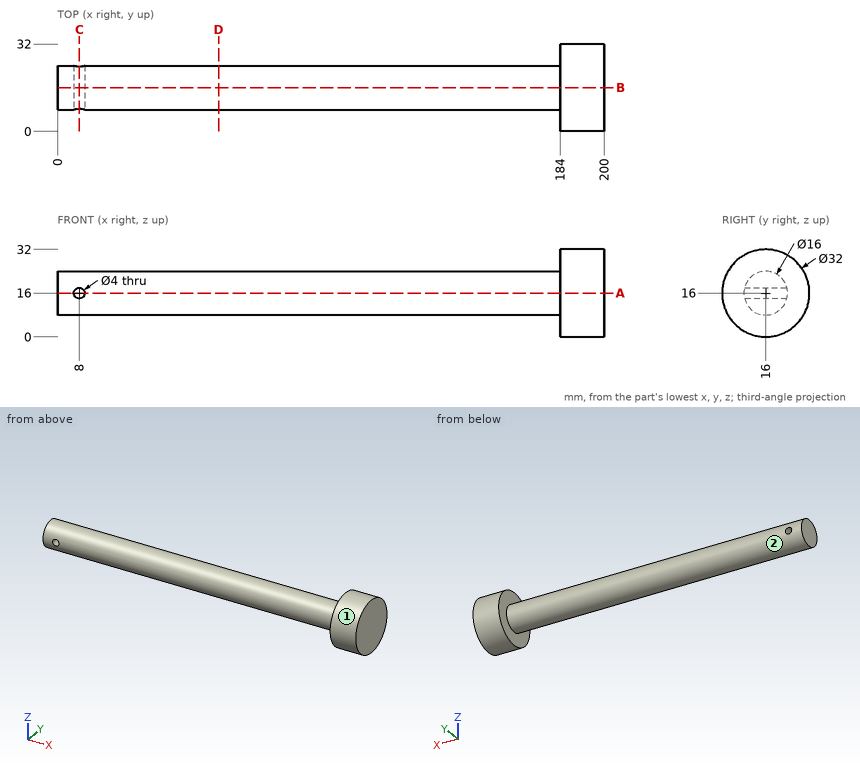
Part print with two shaded views. Sizes in mm from the minimum x, y, z corner. A direction names the side the tool comes from. Coordinates: 2 decimals unless noted, no trailing zeros. Order: outer loops, then holes, each group sorted by start corner. A loop starts at its lowest first (then second) coordinate and runs counter-clockwise, first axis right, second up. Notation, with made-up numbers: (69.25, 30) - (77.25, 30) arc R17 cw to (77.25, 54) - close; hole circle Ø6 at (4, 66). An arc over 180 degrees is marked (long way). Write item = value, one per line. Start each with the question number.
1) Saw through at D-D on x = 59. Write the cut outline in (y, z).
2) Wall check: line 1 along X through (y, z) = (15.75, 16); line 2 along X through (y, z) = (5.5, 23); line 3 along X through (y, z) = (22.5, 14.5). Give the ranges that are in metal, low to high. Write a range as from..to.
3) 3-axis set-ups, long thin cutter, end or side, ignore diameter. For the marked faces 1 and 2: which of +Z, -Z, +X, -X, +Y, -Y reach the whole face in a straight line?
4) Saw through at B-B on y = 16. Write the cut outline in (x, z), then the cut area to 3 significant figures.
5) Saw through at C-C on x = 8. Write the cut outline in (y, z).
6) Flat gauge pins, fed straight in: pin 1 Ø6 at (x, y) = (54.5, 24.5) entering from -Z; pin 2 Ø12 at (x, y) = (72.5, 18.5) entering from -Z; pin 3 Ø12 at (x, z) = (23.5, 20.5) entering from +Y; pin 4 Ø5 at (x, z) = (106, 28) entering from -Y. Where does each tip first touch, or does it go through?
7) Saw through at A-A on z = 16. Write the cut outline in (x, y), then the cut area to 3 significant figures.
From the geometry:
q1.outline = circle Ø16 at (16, 16)
q2.line_1 = 0..6, 10..200
q2.line_2 = 184..200
q2.line_3 = 0..6.68, 9.32..200
q3.face_1 = +X, -X
q3.face_2 = -X
q4.outline = (0, 8) - (184, 8) - (184, 0) - (200, 0) - (200, 32) - (184, 32) - (184, 24) - (0, 24) - close; hole circle Ø4 at (8, 16)
q4.area = 3,440 mm^2
q5.outline = (8.25, 14) arc R8 ccw to (23.75, 14) - close; (8.25, 18) - (23.75, 18) arc R8 ccw to start
q6.pin_1 = 10.19
q6.pin_2 = 8
q6.pin_3 = 24
q6.pin_4 = through
q7.outline = (0, 8) - (6, 8) - (6, 24) - (0, 24) - close; (10, 8) - (184, 8) - (184, 0) - (200, 0) - (200, 32) - (184, 32) - (184, 24) - (10, 24) - close
q7.area = 3,390 mm^2
